Source: CAD feature listing. Evaluate the final solid. Frame: model axes, mm. Give positions to 0.01 mm unless a question says otherwise; leave off trailing zeros. Write each loop counter-clockwise with the first axis right and the second up, starting at its lowest first coordinate (ties: lowest second). Pieces come first, ordered by that corner, then holes. Notation, with made-up numbers: M 46,83.25 L 71,83.25 A26 ccw 71,105.25 Z; hole C 11,-16.75 d6. An arc over 180 degrees is marked long. Return JSON: item names as keys, results as strings.
```python
from build123d import *

# Parameters (mm, degrees)
SKETCH_1_R          = 10.5
SKETCH_1_R_2        = 6.25
EXTRUDE_1_DEPTH     = 13
SKETCH_2_W          = 0.3
SKETCH_2_H          = 50
EXTRUDE_2_DEPTH     = 13
SKETCH_3_R          = 2.5
CUT_EXTRUDE_1_DEPTH = 56.767373974


with BuildPart() as part:
    # 草图1 → 凸台-拉伸1 (new body)
    with BuildSketch(Plane(origin=(0, 0, 0), x_dir=(1, 0, 0), z_dir=(0, 1, 0))):
        with Locations(Location((0, 0, 0), (0, 0, 90))):
            Circle(SKETCH_1_R)
        with Locations(Location((0, 0, 0), (0, 0, 90))):
            Circle(SKETCH_1_R_2, mode=Mode.SUBTRACT)
    extrude(amount=EXTRUDE_1_DEPTH)

    # 草图2 → 凸台-拉伸2 (add)
    with BuildSketch(Plane(origin=(0, 13, 0), x_dir=(1, 0, 0), z_dir=(0, 1, 0))):
        with Locations((10.35, -25)):
            Rectangle(SKETCH_2_W, SKETCH_2_H)
    extrude(amount=-EXTRUDE_2_DEPTH)

    # 草图3 → 切除-拉伸1 (cut, through all)
    with BuildSketch(Plane(origin=(10.5, 0, 0), x_dir=(0, 0, -1), z_dir=(1, 0, 0))):
        with Locations((-45, 6.5)):
            Circle(SKETCH_3_R)
    extrude(amount=-CUT_EXTRUDE_1_DEPTH, mode=Mode.SUBTRACT)


solid = part.part
```
1) Line query: line 1 (X direction, y = 3.5, z = 0); line 2 (Y direction, x = 10.4, z = 45); line 3 (X direction, y = 7, z = 32.5). Output: solid intervals per line, ascending. Write a range as [from, to].
Numbers:
{"line 1": "x = [-10.5, -6.25], [6.25, 10.5]", "line 2": "y = [0, 4], [9, 13]", "line 3": "x = [10.2, 10.5]"}
2) Cut plane A-A, the plane y = 6.5. Return the cut outline in (x, z).
Numbers:
{"outline": "M 10.2,2.49 A10.5 ccw long 10.5,0 L 10.5,42.5 L 10.2,42.5 Z; M 10.2,47.5 L 10.5,47.5 L 10.5,50 L 10.2,50 Z; hole C 0,0 d12.5"}
3) Draft query along X for faces 1 (the face through (-1.88, 6.41, -5.96)), 2 (the face through (10.5, 7, 25)), 3 (the face through (10.35, 5.54, 42.69)). Return one class per face: released by +X, released by -X, zero draft, split by the parting line, or undercut.
Numbers:
{"face 1": "undercut", "face 2": "released by +X", "face 3": "zero draft"}
4) Cut plane C-C, the plane x = 0. Return the cut outline in (y, z), then the cut area to 4 significant figures.
Numbers:
{"outline": "M 0,-10.5 L 13,-10.5 L 13,-6.25 L 0,-6.25 Z; M 0,6.25 L 13,6.25 L 13,10.5 L 0,10.5 Z", "area": "110.5 mm²"}
5) Contact query for flat-ended pins moving along their axis: pin 1 Ø1.5 at (x, y) = (1.5, 3.5) entering from -Z; pin 2 Ø4.5 at (y, z) = (6.5, 45) entering from +X; pin 3 Ø6 at (x, y) = (-8, 9) entering from +Z; pin 4 Ø4 at (x, y) = (8, 7) entering from +Z. Output: stop coordinate, or through.
Numbers:
{"pin 1": "stops at z = -10.47", "pin 2": "passes through", "pin 3": "stops at z = 9.23", "pin 4": "stops at z = 8.62"}
6) Cut plane B-B, the plane z = 45. Return the cut outline in (x, y), then the cut area to 3 significant figures.
Numbers:
{"outline": "M 10.2,0 L 10.5,0 L 10.5,4 L 10.2,4 Z; M 10.2,9 L 10.5,9 L 10.5,13 L 10.2,13 Z", "area": "2.40 mm²"}
7) Cut plane D-D, the plane y = 10.5. Return the cut outline in (x, z), then the cut area to 3 significant figures.
Numbers:
{"outline": "M 10.2,2.49 A10.5 ccw long 10.5,0 L 10.5,50 L 10.2,50 Z; hole C 0,0 d12.5", "area": "238 mm²"}
